Source: CAD feature listing. Evaluate the final solid. Frame: model axes, mm. A direction names the side the tool comes from. Round coordinates to 2 decimals unless told otherwise and drop trailing zeros. Order: outer loops, then holes, each group sorted by start corner. A loop starts at its lowest first (then second) coordinate and runs counter-clockwise, first axis right, second up. Notation, with made-up numbers: M -24.5,61.25 L 1.5,61.25 A26 cw 1.5,97.25 Z; hole C 76.25,-30 d11. An arc over 180 degrees is marked long. Answer as CSV lines item,"result". Start each with the question number.
Item 1: Set-up query: faces 1 (the face through (25, 4, 10)), 2 (the face through (-17, -27, 12)), 3 (the face through (-8.25, -35, 12)), 4 (the face through (25.84, 3.89, 23.19)), 5 (the face through (1.862, 33.126, 16.182)). Return all of +Z, -Z, +X, -X, +Y, -Y with unobstructed straight access to the full face (end or side cutting, diameter ignored); none if empty.
Item 2: Section query B-B on z = 6.5. Return the cut outline in (x, y), plus the area to 3 significant figures.
Item 3: Section query A-A on y = -36. Return the cut outline in (x, z), plus the area to 3 significant figures.
Item 4: Section query C-C on z = 18.75. State how many separate pieces and enclosed holes the cut face has, plus the area to 3 significant figures.
Item 5: Section query D-D on x = 8. Return the cut outline in (y, z).
Item 6: Line query: line 1 (Z direction, x = -9, y = -36); line 2 (Y direction, x = 23, z = 16.5); line 3 (Y direction, x = -17.5, z = 16.25). Output: solid intervals per line, ascending. Write a range as [from, to].
Item 7: Pull-direction query (X, two-part tool) for faces 6 (the face through (15.75, -36, 12)), 7 (the face through (14.23, -39.47, 18.04)), 8 (the face through (20.5, 27, 10)); classes: +X half, -X half, draft (parallel to the pull), parting line (faces both ways), or undercut.
Item 8: First-contact query: P1, Ø8, axis at y = -36, z = 18.5, coming from the -X side; P2, Ø10, axis at x = 20, z = 9.5, coming from the -Y side; P3, Ø6.5, axis at y = -36, z = 18.5, coming from the -X side; P4, Ø1.7, axis at x = 23, z = 9.5, coming from the -Y side. Flat tips, straight axial feed; report the tip coordinate or a pass-through.
from build123d import *

# Parameters (mm, degrees)
BOSS_EXTRUDE1_DEPTH = 25
SKETCH2_R           = 3.5
CUT_EXTRUDE1_DEPTH  = 65.734554142
CUT_EXTRUDE3_REACH  = 96.752
FILLET1_R           = 5


with BuildPart() as part:
    # Sketch1 → Boss-Extrude1 (new body)
    with BuildSketch(Plane.XY):
        Polygon((-20.5, 24), (20.5, 24), (20.5, 31), (25, 31), (25, -24), (12.75, -24), (12.75, -45), (15.75, -45), (15.75, -27), (28, -27), (28, 34), (28, 42), (-23.5, 42), (-23.5, 27), (-23.5, -27), (-11.25, -27), (-11.25, -45), (-8.25, -45), (-8.25, -24), (-20.5, -24), align=None)
    extrude(amount=BOSS_EXTRUDE1_DEPTH)

    # Sketch2 → Cut-Extrude1 (cut, through all)
    with BuildSketch(Plane(origin=(-11.25, 0, 0), x_dir=(0, 0, -1), z_dir=(1, 0, 0))):
        with Locations(Location((-6.5, -36, 0), (0, 0, 270))):
            Circle(SKETCH2_R)
        with Locations(Location((-18.5, -36, 0), (0, 0, 180))):
            Circle(SKETCH2_R)
    extrude(amount=CUT_EXTRUDE1_DEPTH, mode=Mode.SUBTRACT)

    # Cut-Extrude3: up to this face of the body (flat: up to its plane)
    cut_extrude3_end = Plane(part.part.faces().sort_by_distance((0, 24, 12.5))[0])
    # Sketch4 → Cut-Extrude3 (cut, up to the picked face)
    with BuildSketch(Plane(origin=(0, 42, 0), x_dir=(1, 0, 0), z_dir=(0, 1, 0)), mode=Mode.PRIVATE) as cut_extrude3_sk1:
        with BuildLine():
            Line((28, -25), (-23.5, -25))
            ThreePointArc((-23.5, -25), (2.25, -16.180378238), (28, -25))
        make_face()
    cut_extrude3_tool1 = split(extrude(cut_extrude3_sk1.sketch, amount=-CUT_EXTRUDE3_REACH, mode=Mode.PRIVATE), bisect_by=cut_extrude3_end, keep=Keep.BOTH, mode=Mode.PRIVATE)
    add(cut_extrude3_tool1.solids().sort_by(Axis((2.25, 42, 21.438341), (0, -1, 0)))[0], mode=Mode.SUBTRACT)

    # Fillet1
    # the kernel refuses this fillet: 5 mm, written as the material it takes off along each edge
    with BuildSketch(Plane(origin=(25, 35.456439237, 25), x_dir=(0, 0, -1), z_dir=(0, -1, 0))) as fillet1_piece_1_section:
        with BuildLine():
            CenterArc((4.582575695, 5), FILLET1_R, 203.578178478, 66.421821522)
            Line((0, 3), (0, 0))
            Line((0, 0), (4.582575695, 0))
        make_face()
    fillet1_piece_1 = extrude(amount=59.456439237, mode=Mode.PRIVATE)
    fillet1_piece_1 = split(fillet1_piece_1, bisect_by=Plane(origin=(25.306626157, 31, 22.170234041), z_dir=(0, -1, 0)), keep=Keep.TOP, mode=Mode.PRIVATE)
    add(fillet1_piece_1, mode=Mode.SUBTRACT)
    with BuildSketch(Plane(origin=(-20.5, -24, 25), x_dir=(0, 0, -1), z_dir=(0, 1, 0))) as fillet1_piece_2:
        with BuildLine():
            CenterArc((4.582575695, 5), FILLET1_R, 203.578178478, 66.421821522)
            Line((0, 3), (0, 0))
            Line((0, 0), (4.582575695, 0))
        make_face()
    extrude(amount=48, mode=Mode.SUBTRACT)


solid = part.part
Results:
1,face 1,"+Z, -Z"
1,face 2,"+Z, -Z, -X, -Y"
1,face 3,"+Z, -Z, -Y"
1,face 4,"+Z"
1,face 5,"+Z, +Y"
2,outline,"M -23.5,-27 L -11.25,-27 L -11.25,-32.5 L -8.25,-32.5 L -8.25,-24 L -20.5,-24 L -20.5,24 L 20.5,24 L 20.5,31 L 25,31 L 25,-24 L 12.75,-24 L 12.75,-32.5 L 15.75,-32.5 L 15.75,-27 L 28,-27 L 28,42 L -23.5,42 Z; M -11.25,-45 L -8.25,-45 L -8.25,-39.5 L -11.25,-39.5 Z; M 12.75,-45 L 15.75,-45 L 15.75,-39.5 L 12.75,-39.5 Z"
2,area,"1,340 mm^2"
3,outline,"M -11.25,0 L -8.25,0 L -8.25,3 L -11.25,3 Z; M -11.25,10 L -8.25,10 L -8.25,15 L -11.25,15 Z; M -11.25,22 L -8.25,22 L -8.25,25 L -11.25,25 Z; M 12.75,0 L 15.75,0 L 15.75,3 L 12.75,3 Z; M 12.75,10 L 15.75,10 L 15.75,15 L 12.75,15 Z; M 12.75,22 L 15.75,22 L 15.75,25 L 12.75,25 Z"
3,area,"66.0 mm^2"
4,separate pieces,"4"
4,enclosed holes,"0"
4,area,"820 mm^2"
5,outline,"M 24,0 L 42,0 L 42,16.58 L 24,16.58 Z"
6,line 1,"[0, 3], [10, 15], [22, 25]"
6,line 2,"[-27, -24], [31, 42]"
6,line 3,"[-27, -24], [24, 42]"
7,face 6,"+X half"
7,face 7,"draft"
7,face 8,"undercut"
8,P1,"x = -11.25"
8,P2,"y = -45"
8,P3,"through"
8,P4,"y = -27"
